Part model, mm, in its own coordinate system. Give positions to 0.01 mm unless a question says otherwise; leave off trailing zeros. Loops run counter-clockwise (first coordinate to the right, second up) from the corner with the lowest first, then second, coordinate; pieces in that order, holes last. Notation, with made-up numbers: (7.5, 10.25) -> (53.5, 10.25) arc R24 cw to (53.5, 22.25) -> close; hole circle Ø2 at (30, 23). An arc over 180 degrees is marked (long way). One line per question, with ' | ' between items.
Autodesk Fusion 360 part; units mm, degrees
sketch "Sketch1" plane through (0, 0, 0) normal (0, 1, 0) x (1, 0, 0)
  line L0 (0, 0) -> (0, 0.5)
  line L1 (0, 0.5) -> (0.1389, 0.5)
  line L2 (0.1389, 0.5) -> (2.424, 0.5)
  line L3 (0, 0.5) -> (-2.424, 0.5)
  arc A0 (-2.424, 0.5) -> (2.424, 0.5) centre (0, 0) ccw
  dimension "d1" = 4.95
  dimension "d2" = 0.5
extrude "Extrude1" add sketch "Sketch1" along normal blind 3
fillet "Fillet1" radius 0.1 2 edges at (2.424, 1.5, -0.5) (-2.424, 1.5, -0.5)
extrude "Extrude2" add 1 faces at (0, 3, 0.4917) along direction (0, 1, 0) blind 4
1) Saw through at A-A (y = 3.25). Give the cut face in (x, z).
Found:
outline: (-2.44, -0.42) arc R0.1 ccw to (-2.34, -0.5) -> (2.34, -0.5) arc R0.1 ccw to (2.44, -0.42) arc R2.48 ccw (long way) to start
2) Pull direction Y, two halves, no side cores. Call faces 1 (the flat face through (0, 7, 1)), 2 (the flat face through (0, 0, 1)), 3 (the flat face through (0, 3, -0.5)): pulls with the +Y half, pulls with the -Y half, needs draft (parallel to the pull), parting line crosses it, or undercut.
Found:
face 1: pulls with the +Y half | face 2: pulls with the -Y half | face 3: needs draft
3) Drill centre lines: line 1 (Z direction, x = 0.4, y = 5); line 2 (Z direction, x = -0.25, y = 3.75); line 3 (X direction, y = 4.75, z = 2.25). Where is each one in solid material? Low to high.
Found:
line 1: -0.5 to 2.44 | line 2: -0.5 to 2.46 | line 3: -1.03 to 1.03
4) Saw through at B-B (x = -1.65). Give the cut face in (y, z).
Found:
outline: (0, -0.5) -> (7, -0.5) -> (7, 1.84) -> (0, 1.84) -> close
